from build123d import *

# Parameters (mm, degrees)
BOSS_EXTRUDE2_DEPTH         = 25
SKETCH2_R                   = 5
CUT_EXTRUDE1_DEPTH          = 63
CUT_EXTRUDE2_DEPTH          = 10
SKETCH4_R                   = 12.5
BOSS_EXTRUDE4_DEPTH         = 10
SKETCH10_R                  = 10
CUT_EXTRUDE3_DEPTH          = 15
SKETCH11_R                  = 5
CUT_EXTRUDE4_DEPTH          = 872
CUT_EXTRUDE6_DEPTH          = 10
M12X1_25_TAPPED_HOLE1_D     = 10.8
M12X1_25_TAPPED_HOLE1_DEPTH = 15
M12X1_25_TAPPED_HOLE1_TIP   = 3.244647343


with BuildPart() as part:
    # Sketch1 → Boss-Extrude2 (new body)
    with BuildSketch(Plane.XY):
        with BuildLine():
            Line((-45, -5), (-20, 20))
            Line((-20, 20), (0, 0))
            Line((0, 0), (-25, -25))
            ThreePointArc((-25, -25), (-32.004902432, -30.742646352), (-40, -35))
            Line((-40, -35), (-70, -35))
            ThreePointArc((-70, -35), (-85, -20), (-70, -5))
            Line((-70, -5), (-45, -5))
        make_face()
    extrude(amount=BOSS_EXTRUDE2_DEPTH)

    # Sketch2 → Cut-Extrude1 (cut)
    with BuildSketch(Plane.XY.offset(25)):
        with Locations((-20, 0)):
            Circle(SKETCH2_R)
    extrude(amount=-CUT_EXTRUDE1_DEPTH, mode=Mode.SUBTRACT)

    # Sketch3 → Cut-Extrude2 (cut)
    with BuildSketch(Plane.XY.offset(25)):
        with BuildLine():
            Line((-6.464921114, 6.464921114), (-13.535078886, 13.535078886))
            Line((-13.535078886, 13.535078886), (-23.478357909, 3.591799863))
            ThreePointArc((-23.478357909, 3.591799863), (-18.049588447, 4.603899953), (-15, 0))
            ThreePointArc((-15, 0), (-15.365401888, -1.876299641), (-16.408200137, -3.478357909))
            Line((-16.408200137, -3.478357909), (-6.464921114, 6.464921114))
        make_face()
    extrude(amount=-CUT_EXTRUDE2_DEPTH, mode=Mode.SUBTRACT)

    # Sketch4 → Boss-Extrude4 (add)
    with BuildSketch(Plane.XY.offset(25)):
        with Locations((-40, -20)):
            Circle(SKETCH4_R)
    extrude(amount=BOSS_EXTRUDE4_DEPTH)

    # Sketch10 → Cut-Extrude3 (cut)
    with BuildSketch(Plane.XY.offset(25)):
        with Locations((-70, -20)):
            Circle(SKETCH10_R)
    extrude(amount=-CUT_EXTRUDE3_DEPTH, mode=Mode.SUBTRACT)

    # Sketch11 → Cut-Extrude4 (cut)
    with BuildSketch(Plane.XY.offset(10)):
        with Locations((-70, -20)):
            Circle(SKETCH11_R)
    extrude(amount=-CUT_EXTRUDE4_DEPTH, mode=Mode.SUBTRACT)

    # Sketch12 → Cut-Extrude6 (cut)
    with BuildSketch(Plane.XY.offset(25)):
        with BuildLine():
            Line((-70, -30), (-81.180339887, -30))
            ThreePointArc((-81.180339887, -30), (-85, -20), (-81.180339887, -10))
            Line((-81.180339887, -10), (-70, -10))
            ThreePointArc((-70, -10), (-80, -20), (-70, -30))
        make_face()
    extrude(amount=-CUT_EXTRUDE6_DEPTH, mode=Mode.SUBTRACT)

    # M12x1.25 Tapped Hole1
    with Locations(Plane.XY.offset(35)):
        with Locations((-40, -20)):
            Hole(M12X1_25_TAPPED_HOLE1_D / 2, depth=M12X1_25_TAPPED_HOLE1_DEPTH)
            with Locations((0, 0, -(M12X1_25_TAPPED_HOLE1_DEPTH + M12X1_25_TAPPED_HOLE1_TIP / 2))):  # 118° drill point
                Cone(0, M12X1_25_TAPPED_HOLE1_D / 2, M12X1_25_TAPPED_HOLE1_TIP, mode=Mode.SUBTRACT)


solid = part.part
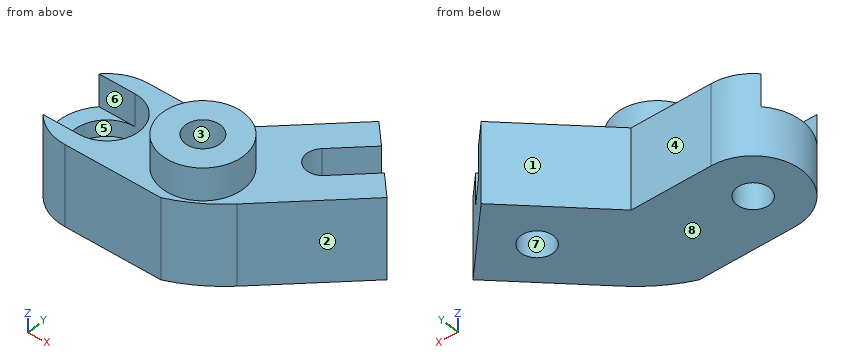
Geometry check sheet. Reference: the model listing, model coordinates, mm. Face numbers are marked on the shaded views. A direction names the side the tool comes from. Give positions to 0.01 mm unless a question says otherwise; leave off trailing zeros. Loops run counter-clockwise (first coordinate to the right, second up) from the corner with the lowest first, then second, coordinate; pieces in that order, holes last.
(1) Section check B-B on y = 2.5. Record the cut outline in (x, z).
From the geometry:
outline: (-37.5, 0) - (-24.33, 0) - (-24.33, 25) - (-37.5, 25) - close; (-15.67, 0) - (-2.5, 0) - (-2.5, 25) - (-10.43, 25) - (-10.43, 15) - (-15.67, 15) - close
(2) Section check C-C on x = -28.5. Record the cut outline in (y, z).
From the geometry:
outline: (-28.16, 0) - (11.5, 0) - (11.5, 25) - (-15.1, 25) - (-15.1, 35) - (-24.9, 35) - (-24.9, 25) - (-28.16, 25) - close
(3) Depth check by flat-ended pin: pin 1 Ø17.5 at (x, y) = (-40, -20) entering from -Z; pin 2 Ø10 at (x, y) = (-53.5, -1.5) entering from +Z; pin 3 Ø16 at (x, y) = (-69.5, -21.5) entering from +Z; pin 4 Ø4.5 at (x, y) = (-78, -23) entering from +Z. Enter the tip coordinate at first touch or a pass-through.
From the geometry:
pin 1: stops at z = 0
pin 2: stops at z = 25
pin 3: stops at z = 10
pin 4: stops at z = 15
(4) Thickness scan on L1, parallel to X at y = 0, z = 6.75; L2, parallel to Y at x = -70, z = 20; L3, parallel to Y at x = -40, z = 31. Record the ranges inside material, lowest first.
From the geometry:
L1: x = -40 to -25, -15 to 0
L2: y = -35 to -30, -10 to -5
L3: y = -32.5 to -25.4, -14.6 to -7.5
(5) Section check D-D on y = -31. Record the cut outline in (x, z).
From the geometry:
outline: (-80.2, 0) - (-32.4, 0) - (-32.4, 25) - (-34.06, 25) - (-34.06, 35) - (-45.94, 35) - (-45.94, 25) - (-80.2, 25) - close
(6) Section check A-A on z = 13. Record the cut outline in (x, y), then the cut area to 3 significant figures.
From the geometry:
outline: (-70, -35) - (-40, -35) arc R45.96 ccw to (-25, -25) - (0, 0) - (-20, 20) - (-45, -5) - (-70, -5) arc R15 ccw to start; hole circle Ø20 at (-70, -20); hole circle Ø10 at (-20, 0)
area: 2,050 mm2
(7) Release check for a two-part mould opening along Y. For the marked faces 1, 2 and 3 record: released by +Y, released by -Y, zero draft, split by the parting line, or undercut.
From the geometry:
face 1: released by +Y
face 2: released by -Y
face 3: undercut
(8) Set-up check for the marked faces 4, 5, 6, 7 and 8: record each of +Z, -Z, +X, -X, +Y, -Y from which the full face is reachable in a straight line by a thin tool's end or side.
From the geometry:
face 4: +Z, -Z, -X, +Y
face 5: +Z
face 6: +Z, -X
face 7: +Z, -Z
face 8: -Z, +X, -X, +Y, -Y
